Here's how the part is built. I have some questions about the finished solid (model axes, mm). A direction names the side the tool comes from. Give positions to 0.01 mm unless a question says otherwise; leave off trailing zeros. Loops run counter-clockwise (first coordinate to the right, second up) from the corner with the lowest first, then second, coordinate; pieces in that order, holes last.
Q1. Thinking about a two-plate mould opening in X: for faces 1 (the face through (-32.215, 72.958, -7.154)), 2 (the face through (2.27, 37.47, -1.89)), 3 (the face through (-2.793, 37.468, -2.864)), 4 (the face through (-7, 76, 0)), which applies, pulls with the +X half, pulls with the -X half, needs draft (parallel to the pull), parting line crosses it, or undercut?
Q2. Suppose I cut it at B-B (x = 15). List the corners of the cut face in (y, z) for me.
Q3. Suppose I cut it at A-A (y = 67). List the corners of the cut face in (x, z) for me.
Q4. Suppose I cut it at D-D (z = 20). List the corners of the cut face in (x, y) for me.
Q5. Suppose I cut it at C-C (z = -1). List the corners of the cut face in (x, y) for me, and give its area (3 significant figures).
Q6. I need wall thicknesses on probe 1 along Z at (x, y) = (-10, 41.5); probe 2 along X at (y, z) = (26, -13.5); probe 3 along X at (y, z) = (54.5, 0). Which ranges of each line are inside material? Lowest first, please.
Q7. I'm going to push flat-ended pins straight in: P1, Ø1, axis at x = 18, y = 53.5, coming from the +Z side; P2, Ø2, axis at x = 20, y = 49, coming from the -Z side; P3, Ø4, axis at x = 7.5, y = 48, coming from the +Z side. Where does each tip first touch, or does it pass through?
Q8. For faces 5 (the face through (0, 0, 6)), 6 (the face through (-27, 70, -7)), 7 (the face through (2.21, 37.47, 2.26)), which set-ups out of +Z, -Z, +X, -X, +Y, -Y let a thin tool reach every point of the face, with its end or its side?
```python
from build123d import *

# Parameters (mm, degrees)
SKETCH2_R           = 27.6
BOSS_EXTRUDE1_DEPTH = 70
CUT_EXTRUDE1_DEPTH  = 50
SKETCH3_R           = 2.75
CUT_EXTRUDE2_DEPTH  = 110
SKETCH4_R           = 33
BOSS_EXTRUDE2_DEPTH = 6
CUT_EXTRUDE3_START  = 6
SKETCH3_2_R         = 2.75
CUT_EXTRUDE3_DEPTH  = 6
CUT_EXTRUDE4_DEPTH  = 81


with BuildPart() as part:
    # Sketch2 → Boss-Extrude1 (new body)
    with BuildSketch(Plane(origin=(0, 0, 0), x_dir=(1, 0, 0), z_dir=(0, 1, 0))):
        with Locations(Location((0, 0, 0), (0, 0, 270))):
            Circle(SKETCH2_R)
    extrude(amount=BOSS_EXTRUDE1_DEPTH)

    # Sketch2_4 → Cut-Extrude1 (cut)
    with BuildSketch(Plane(origin=(0, 0, 0), x_dir=(1, 0, 0), z_dir=(0, 1, 0))):
        with BuildLine():
            Line((-3.997017731, -0.154432059), (0.158545764, -4.309995554))
            Line((0.158545764, -4.309995554), (4.314106781, -0.154434537))
            Line((4.314106781, -0.154434537), (0.162994526, 3.996677718))
            ThreePointArc((0.162994526, 3.996677718), (-2.825395827, 2.831455177), (-3.997017731, -0.154432059))
        make_face()
    extrude(amount=CUT_EXTRUDE1_DEPTH, mode=Mode.SUBTRACT)

    # Sketch3 → Cut-Extrude2 (cut)
    with BuildSketch(Plane(origin=(0, 70, 0), x_dir=(1, 0, 0), z_dir=(0, 1, 0))):
        with Locations(Location((-8.28675, 14.35307203, 0), (0, 0, 270))):
            Circle(SKETCH3_R)
        with Locations(Location((-16.5735, 0, 0), (0, 0, 270))):
            Circle(SKETCH3_R)
        with Locations(Location((-8.28675, -14.35307203, 0), (0, 0, 270))):
            Circle(SKETCH3_R)
        with Locations(Location((8.28675, -14.35307203, 0), (0, 0, 270))):
            Circle(SKETCH3_R)
        with Locations(Location((16.5735, 0, 0), (0, 0, 270))):
            Circle(SKETCH3_R)
        with Locations(Location((8.28675, 14.35307203, 0), (0, 0, 270))):
            Circle(SKETCH3_R)
    extrude(amount=-CUT_EXTRUDE2_DEPTH, mode=Mode.SUBTRACT)

    # Sketch4 → Boss-Extrude2 (add)
    with BuildSketch(Plane(origin=(0, 70, 0), x_dir=(1, 0, 0), z_dir=(0, 1, 0))):
        with Locations(Location((0, 0, 0), (0, 0, 270))):
            Circle(SKETCH4_R)
    extrude(amount=BOSS_EXTRUDE2_DEPTH)

    # Sketch3_2 → Cut-Extrude3 (cut)
    with BuildSketch(Plane(origin=(0, 70, 0), x_dir=(1, 0, 0), z_dir=(0, 1, 0)).offset(CUT_EXTRUDE3_START)):
        with Locations(Location((-8.28675, 14.35307203, 0), (0, 0, 270))):
            Circle(SKETCH3_2_R)
        with Locations(Location((-16.5735, 0, 0), (0, 0, 270))):
            Circle(SKETCH3_2_R)
        with Locations(Location((-8.28675, -14.35307203, 0), (0, 0, 270))):
            Circle(SKETCH3_2_R)
        with Locations(Location((8.28675, -14.35307203, 0), (0, 0, 270))):
            Circle(SKETCH3_2_R)
        with Locations(Location((16.5735, 0, 0), (0, 0, 270))):
            Circle(SKETCH3_2_R)
        with Locations(Location((8.28675, 14.35307203, 0), (0, 0, 270))):
            Circle(SKETCH3_2_R)
    extrude(amount=-CUT_EXTRUDE3_DEPTH, mode=Mode.SUBTRACT)

    # Sketch2_5 → Cut-Extrude4 (cut)
    with BuildSketch(Plane(origin=(0, 0, 0), x_dir=(1, 0, 0), z_dir=(0, 1, 0))):
        with BuildLine():
            Line((-3.997017731, -0.154432059), (0.158545764, -4.309995554))
            Line((0.158545764, -4.309995554), (4.314106781, -0.154434537))
            Line((4.314106781, -0.154434537), (0.162994526, 3.996677718))
            ThreePointArc((0.162994526, 3.996677718), (-2.825395827, 2.831455177), (-3.997017731, -0.154432059))
        make_face()
    extrude(amount=CUT_EXTRUDE4_DEPTH, mode=Mode.SUBTRACT)


solid = part.part
```
Solutions:
1. face 1: parting line crosses it
1. face 2: undercut
1. face 3: undercut
1. face 4: needs draft
2. outline: (0, -23.17) - (70, -23.17) - (70, -29.39) - (76, -29.39) - (76, -2.26) - (0, -2.26) - close; (0, 2.26) - (76, 2.26) - (76, 29.39) - (70, 29.39) - (70, 23.17) - (0, 23.17) - close
3. outline: circle Ø55.2 at (0, 0); hole circle Ø5.5 at (-16.57, 0); hole circle Ø5.5 at (-8.29, -14.35); hole circle Ø5.5 at (-8.29, 14.35); hole (-4, 0.15) arc R4 ccw to (0.16, -4) - (4.31, 0.15) - (0.16, 4.31) - close; hole circle Ø5.5 at (8.29, -14.35); hole circle Ø5.5 at (8.29, 14.35); hole circle Ø5.5 at (16.57, 0)
4. outline: (-26.25, 70) - (-19.02, 70) - (-19.02, 0) - (19.02, 0) - (19.02, 70) - (26.25, 70) - (26.25, 76) - (-26.25, 76) - close
5. outline: (-32.98, 70) - (-27.58, 70) - (-27.58, 0) - (-19.14, 0) - (-19.14, 76) - (-32.98, 76) - close; (-14.01, 0) - (-3.87, 0) - (-3.87, 76) - (-14.01, 76) - close; (3.16, 0) - (14.01, 0) - (14.01, 76) - (3.16, 76) - close; (19.14, 0) - (27.58, 0) - (27.58, 70) - (32.98, 70) - (32.98, 76) - (19.14, 76) - close
5. area: 2,940 mm2
6. probe 1: z = -25.72 to -16.5, -12.2 to 12.2, 16.5 to 25.72
6. probe 2: x = -24.07 to -10.9, -5.67 to 5.67, 10.9 to 24.07
6. probe 3: x = -27.6 to -19.32, -13.82 to -4, 4.16 to 13.82, 19.32 to 27.6
7. P1: stops at z = 21.34
7. P2: stops at z = -20.02
7. P3: stops at z = 27.05
8. face 5: +Z, -Z, +X, -X, -Y
8. face 6: -Y
8. face 7: +Y, -Y
